CAD build for the part. Positions are in the model's coordinates, mm. Face numbers are marked on the shaded views. Give positions to 0.01 mm unless a question says otherwise; leave off trailing zeros. Order: outer loops, then holes, each group sorted by start corner. A loop starts at its lowest first (then second) coordinate and runs counter-clockwise, first axis right, second up.
Autodesk Inventor part; units mm, degrees
ref_plane "YZ Plane" through (0, 0, 0) normal (1, 0, 0) x (0, 1, 0)
ref_plane "XZ Plane" through (0, 0, 0) normal (0, 1, 0) x (-1, 0, 0)
ref_plane "XY Plane" through (0, 0, 0) normal (0, 0, 1) x (1, 0, 0)
sketch "Sketch1" plane through (0, 0, 0) normal (0, 0, 1) x (1, 0, 0)
  line L0 (-50, -100) -> (50, -100)
  line L1 (50, -100) -> (50, 100)
  line L2 (50, 100) -> (-50, 100)
  line L3 (-50, 100) -> (-50, -100)
  line L4 (-50, -100) -> (50, 100) construction
  line L5 (50, -100) -> (-50, 100) construction
  point P0 (0, 0)
  dimension "d0" = 100
  dimension "d1" = 200
extrude "Extrusion1" add sketch "Sketch1" along normal blind 5
sketch "Sketch6" plane through (0, 0, 5) normal (0, 0, 1) x (1, 0, 0)
  line L0 (4.9986, 75) -> (-5.0014, 75)
  line L1 (-25.0014, 55) -> (-25.0014, 45)
  line L2 (-5.0014, 25) -> (4.9986, 25)
  line L3 (24.9986, 45) -> (24.9986, 55)
  line L4 (24.9986, 75) -> (-25.0014, 25) construction
  line L5 (-25.0014, 75) -> (24.9986, 25) construction
  arc A0 (4.9986, 25) -> (24.9986, 45) centre (4.9986, 45) ccw
  arc A1 (24.9986, 55) -> (4.9986, 75) centre (4.9986, 55) ccw
  arc A2 (-5.0014, 75) -> (-25.0014, 55) centre (-5.0014, 55) ccw
  arc A3 (-25.0014, 45) -> (-5.0014, 25) centre (-5.0014, 45) ccw
  point P0 (0, 0)
  point P1 (-0.0014, 50)
  dimension "d21" = 50
  dimension "d22" = 50
  dimension "d23" = 20
extrude "Extrusion6" cut sketch "Sketch6" against normal blind 5
sketch "Sketch15" plane through (-50, 100, 5) normal (0, 1, 0) x (1, 0, 0)
  line L0 (100, 0) -> (0, 0)
  line L1 (0, 0) -> (100, 0)
  line L2 (100, 0) -> (100, 30)
  line L3 (100, 30) -> (0, 30)
  line L4 (0, 30) -> (0, 0)
  point P0 (50, 5)
  dimension "d46" = 100
  dimension "d47" = 30
sketch "Sketch16" plane through (-50, 100, 5) normal (0, 1, 0) x (1, 0, 0)
  circle A0 centre (10.5, 5) radius 4.5
  circle A1 centre (89.5, 5) radius 4.5
  circle A2 centre (10.5, 25) radius 4.5
  circle A3 centre (89.5, 25) radius 4.5
  point P0 (50, 5)
  dimension "d48" = 9
  dimension "d49" = 9
  dimension "d50" = 9
  dimension "d51" = 9
extrude "Extrusion11" add sketch "Sketch15" against normal blind 5
extrude "Extrusion12" add sketch "Sketch16" along normal blind 15
sketch "Sketch17" plane through (50, 100, -25) normal (0, 0, -1) x (-1, 0, 0)
  line L0 (100.0829, 0) -> (0.0829, 0)
  line L1 (0.0829, 0) -> (0.0829, -30)
  line L2 (0.0829, -30) -> (100.0829, -30)
  line L3 (100.0829, -30) -> (100.0829, 0)
  point P0 (50, -100)
  dimension "d56" = 100
  dimension "d57" = 30
extrude "Extrusion13" add sketch "Sketch17" against normal blind 5
sketch "Sketch18" plane through (49.9171, 70, -25) normal (1, 0, 0) x (0, 0, -1)
  line L0 (0, 0) -> (-5, 0)
  line L1 (-30, 30) -> (-30, -170)
  line L2 (0, 0) -> (-30, 0)
  line L3 (-30, 0) -> (-30, 30)
  line L4 (-30, 30) -> (0, 30)
  line L5 (0, 30) -> (0, 0)
  point P0 (-25, -70)
extrude "Extrusion14" add sketch "Sketch18" against normal blind 5
sketch "Sketch20" plane through (-50, -100, 5) normal (-1, 0, 0) x (0, 0, 1)
  line L0 (-30, 200) -> (0, 200)
  line L1 (-30, 170) -> (-30, 200)
  line L2 (0, 200) -> (-30, 200)
  line L3 (-30, 200) -> (-30, 170)
  line L4 (-30, 170) -> (0, 170)
  line L5 (0, 170) -> (0, 200)
  point P0 (-5, 100)
extrude "Extrusion16" add sketch "Sketch20" against normal blind 5
properties part number "fixation_v02"
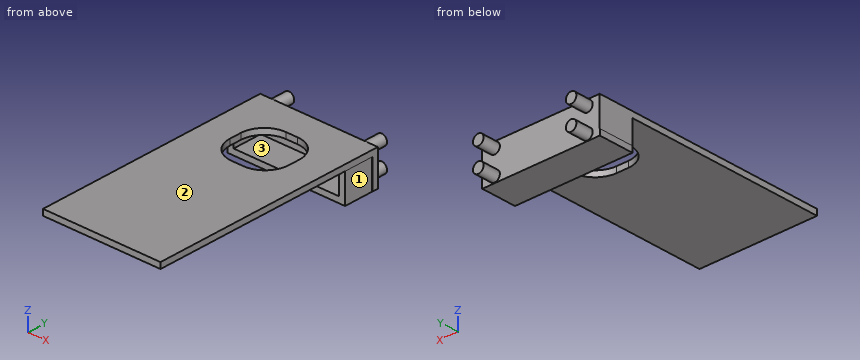
Item 1: Slice it at A-A (z = -12.25). Give the cut face in (x, y).
Item 2: Slice it at B-B (x = -39.5). Give the cut face in (y, z).
Item 3: Slice it at D-D (x = -28). Give the cut face in (y, z), and give its area (3 significant figures).
Item 4: Slice it at C-C (y = 17). Give the cut face in (x, z).
Item 5: Drop flat-ended pins along their axis: pin 1 Ø8 at (x, z) = (2.5, -8) entering from +Y; pin 2 Ø10 at (x, z) = (15.5, -9.5) entering from -Y; pin 3 Ø1.5 at (y, z) = (51, 3) entering from -X. Give the stop position or say it passes through.
Item 6: Two-plate mould, pull along Z, no slides. Class the marked faces 1, 2 and 3: released by +Z, released by -Z, zero draft, split by the parting line, or undercut.
Item 7: Wall check: L1, parallel to Z at x = 37, y = 85; L2, parallel to X at y = 74.5, z = -1.75; L3, parallel to Z at x = 4, y = -41.5. Give the ranges that are in metal, low to high.
A:
1. outline: (-50, 70) - (-45, 70) - (-45, 95) - (44.92, 95) - (44.92, 70) - (49.92, 70) - (49.92, 95) - (50, 95) - (50, 100) - (-50, 100) - close
2. outline: (-100, 0) - (95, 0) - (95, -20) - (70, -20) - (70, -25) - (100, -25) - (100, -24.5) - (115, -24.5) - (115, -15.5) - (100, -15.5) - (100, -4.5) - (115, -4.5) - (115, 4.5) - (100, 4.5) - (100, 5) - (-100, 5) - close
3. outline: (-100, 0) - (95, 0) - (95, -20) - (70, -20) - (70, -25) - (100, -25) - (100, 5) - (-100, 5) - close
3. area: 1,250 mm2
4. outline: (-50, 0) - (50, 0) - (50, 5) - (-50, 5) - close
5. pin 1: stops at y = 100
5. pin 2: stops at y = 95
5. pin 3: stops at x = -50
6. face 1: zero draft
6. face 2: released by +Z
6. face 3: undercut
7. L1: z = -25 to -20, 0 to 5
7. L2: x = -50 to -45, 44.92 to 49.92
7. L3: z = 0 to 5
